Geometry: see drawing. Coordinates: mm, zero at the bounding-box minimum. Coordinates: 2 decimals unless noted, no trailing zeros. Order: outer loops, then holes, each group sorted by start corner. A loop starts at its lowest first (then second) coordinate and runs counter-clockwise, first axis right, second up. Notation, with made-up numbers: (-29, -30.75) -> (9, -30.75) arc R17 ccw to (9, -24.75) -> close; hole circle Ø4 at (7.5, 38). An arc over 180 degrees is marked (long way). Write each question's results on one line, items separated by ' | '. Start each with the question number.
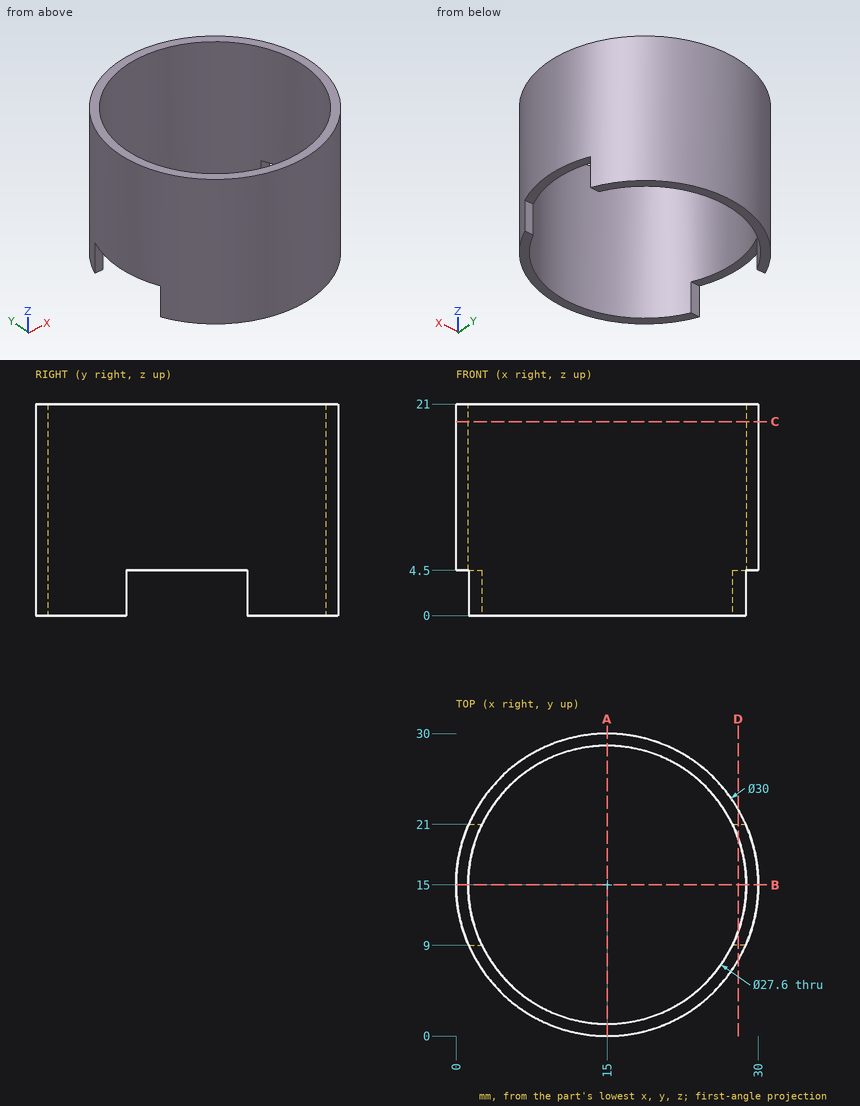
(1) Section A-A on x = 15. Return the cut outline in (y, z), then the cut area to 3 significant figures.
(2) Line query: L1, parallel to X at y = 15.25, z = 13; L2, parallel to X at y = 19.25, z = 13.5. Output: solid intervals per line, ascending.
(3) Section D-D on x = 28. Return the cut outline in (y, z), then the cut area to 3 significant figures.
(4) First-contact query: P1, Ø6, axis at x = 24.5, y = 18, coming from the +Z side; P2, Ø2, axis at y = 10.5, z = 5, coming from the -X side; P3, Ø1.1, axis at x = 2, z = 1.5, coming from the -Y side; P4, Ø3, axis at x = 0.5, y = 16, coming from the -Z side. Flat tips, straight axial feed; report the tip coordinate or a pass-through.
(5) Section C-C on z = 19.25. Return the cut outline in (x, y).
(6) Section B-B on y = 15. Return the cut outline in (x, z), then the cut area to 3 significant figures.
Results list:
1) outline: (0, 0) -> (1.2, 0) -> (1.2, 21) -> (0, 21) -> close; (28.8, 0) -> (30, 0) -> (30, 21) -> (28.8, 21) -> close | area: 50.4 mm²
2) L1: x = 0 to 1.2, 28.8 to 30 | L2: x = 0.61 to 1.87, 28.13 to 29.39
3) outline: (7.52, 0) -> (9, 0) -> (9, 4.5) -> (10.37, 4.5) -> (10.37, 21) -> (7.52, 21) -> close; (19.63, 4.5) -> (21, 4.5) -> (21, 0) -> (22.48, 0) -> (22.48, 21) -> (19.63, 21) -> close | area: 107 mm²
4) P1: passes through | P2: stops at x = 0.41 | P3: stops at y = 6.63 | P4: stops at z = 4.5
5) outline: circle Ø30 at (15, 15); hole circle Ø27.6 at (15, 15)
6) outline: (0, 4.5) -> (1.2, 4.5) -> (1.2, 21) -> (0, 21) -> close; (28.8, 4.5) -> (30, 4.5) -> (30, 21) -> (28.8, 21) -> close | area: 39.6 mm²
